Verification items for the finished model (mm, model axes). Give positions to 0.01 mm unless a question says otherwise; leave off trailing zeros. Order: outer loops, then holes, each group sorted by start corner. A loop starts at its lowest first (then second) coordinate and runs counter-clockwise, first axis right, second up.
(1) Sectioned sample at C-C on z = -1.75. Record the cut outline in (x, y), plus the area to 3 significant figures.
(2) Sectioned sample at A-A on x = -25.5. Record the cut outline in (y, z), plus the area to 3 significant figures.
(3) Gauge pin test, flat ends, axial feed: pin 1 (2 mm diameter, centred on y = 21.5, z = -2, fed in from +X); pin 2 (2 mm diameter, centred on y = 32, z = -2, fed in from +X). Record the tip position at first contact, or that the pin passes through.
(4) Sectioned sample at B-B on y = 15.5. Record the cut outline in (x, z).
(5) Mould release check, pull along X, two halves, no side actions. Record for faces 1 (the face through (3.96, 41.86, -2.32)), 2 (the face through (-33.024, 19.349, -2.254)), 3 (the face through (6, 31, 0)): pulls with the +X half, pulls with the -X half, needs draft (parallel to the pull), parting line crosses it, or undercut.
(6) Scan lines: L1, parallel to X at y = 42.5, z = -1.85; L2, parallel to X at y = 38, z = -1.3; L3, parallel to Y at x = -21.5, z = -2.2. Record each from-to range of solid material in increasing order.
(7) Sectioned sample at D-D on y = 52.5. Record the cut outline in (x, z), plus the area to 3 significant figures.
```python
from build123d import *

# Parameters (mm, degrees)
SKETCH1_R             = 7.178016374
EXTRUDE1_DEPTH        = 4.572
CIRPATTERN3_START     = -4.572
CIRPATTERN3_OUTLINE_R = 7.178016374
CIRPATTERN3_DEPTH     = 4.572


# Read off the part's stored shape, not the designer's step: CirPattern3
with BuildPart() as part:
    # Sketch1 → Extrude1 (new body)
    with BuildSketch(Plane.XY):
        with BuildLine():
            Line((-17.82605161, 0), (61.168535359, 0))
            ThreePointArc((61.168535359, 0), (20.218554782, 57.730405857), (-47.802514574, 38.164241357))
            Line((-47.802514574, 38.164241357), (-17.82605161, 0))
        make_face()
        with Locations((37.24834288, 21.505340789)):
            Circle(SKETCH1_R, mode=Mode.SUBTRACT)
    extrude(amount=-EXTRUDE1_DEPTH)

    # CirPattern3 outline → CirPattern3 (cut)
    with BuildSketch(Plane.XY.offset(CIRPATTERN3_START)):
        with Locations((-21.505340789, 37.24834288)):
            Circle(CIRPATTERN3_OUTLINE_R)
        with Locations((11.131983535, 41.545128142)):
            Circle(CIRPATTERN3_OUTLINE_R)
    extrude(amount=CIRPATTERN3_DEPTH, mode=Mode.SUBTRACT)


solid = part.part
```
Ans:
1. outline: (-47.8, 38.16) - (-17.83, 0) - (61.17, 0) arc R61.17 ccw to start; hole circle Ø14.36 at (-21.51, 37.25); hole circle Ø14.36 at (11.13, 41.55); hole circle Ø14.36 at (37.25, 21.51)
1. area: 4,470 mm2
2. outline: (9.77, -4.57) - (31.28, -4.57) - (31.28, 0) - (9.77, 0) - close; (43.21, -4.57) - (55.6, -4.57) - (55.6, 0) - (43.21, 0) - close
2. area: 155 mm2
3. pin 1: stops at x = 57.63
3. pin 2: stops at x = 52.73
4. outline: (-30, -4.57) - (33.32, -4.57) - (33.32, 0) - (-30, 0) - close; (41.18, -4.57) - (59.17, -4.57) - (59.17, 0) - (41.18, 0) - close
5. face 1: undercut
5. face 2: pulls with the -X half
5. face 3: needs draft
6. L1: x = -43.99 to -26.4, -16.61 to 4.02, 18.25 to 43.99
6. L2: x = -47.67 to -28.64, -14.37 to 4.89, 17.37 to 47.93
6. L3: y = 4.68 to 30.07, 44.43 to 57.27
7. outline: (-31.39, -4.57) - (31.39, -4.57) - (31.39, 0) - (-31.39, 0) - close
7. area: 287 mm2
